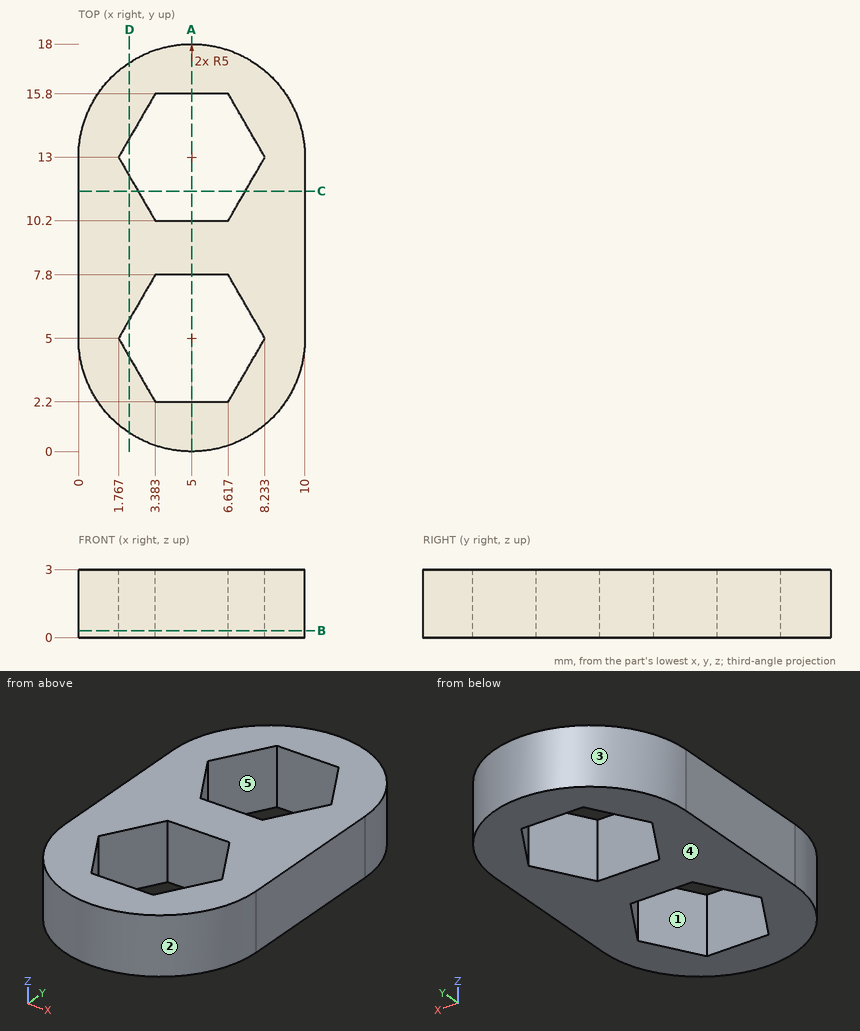
Geometry: see drawing. Coordinates: mm, zero at the bounding-box minimum. A direction names the side the tool comes from. Give positions to 0.01 mm unless a question says otherwise; leave off trailing zeros. Order: outer loops, then holes, each group sorted by start corner. A loop starts at its lowest first (then second) coordinate and runs counter-clockwise, first axis right, second up. Notation, with made-up numbers: (1, -9) -> (15, -9) arc R5 ccw to (15, 0) -> close; hole circle Ø9 at (-11.75, -2). An arc over 180 degrees is marked (long way). Write each question's results on one line, items separated by ' | '. Start each with the question number.
1) Line query: line 1 (Y direction, x = 5.75, z = 2.3); line 2 (Y direction, x = 6.75, z = 1.6) (1 decimal); line 3 (X direction, y = 4.5, z = 1.2) (1 decimal). Output: solid intervals per line, ascending. Write a range as from..to.
2) Draft query along Y for the marked faces 3, 4 and 5. Return one class per face: pulls with the +Y half, pulls with the -Y half, needs draft (parallel to the pull), parting line crosses it, or undercut.
3) Set-up query: the marked faces 1 and 2. Return all of +Z, -Z, +X, -X, +Y, -Y with unobstructed straight access to the full face (end or side cutting, diameter ignored); none if empty.
4) Section A-A (x = 5). Return loops of the section in (y, z).
5) Section B-B (z = 0.3). Return loops of the section in (x, y), then the cut area to 3 significant figures.
6) Section C-C (y = 11.5). Return loops of the section in (x, z).
7) Section D-D (x = 2.25). Return loops of the section in (y, z) (1 decimal), then the cut area to 3 significant figures.
Calculated:
1) line 1: 0.06..2.2, 7.8..10.2, 15.8..17.94 | line 2: 0.3..2.4, 7.6..10.4, 15.6..17.7 | line 3: 0..2.1, 7.9..10
2) face 3: pulls with the +Y half | face 4: needs draft | face 5: undercut
3) face 1: +Z, -Z | face 2: +Z, -Z, -Y
4) outline: (0, 0) -> (2.2, 0) -> (2.2, 3) -> (0, 3) -> close; (7.8, 0) -> (10.2, 0) -> (10.2, 3) -> (7.8, 3) -> close; (15.8, 0) -> (18, 0) -> (18, 3) -> (15.8, 3) -> close
5) outline: (0, 5) arc R5 ccw to (10, 5) -> (10, 13) arc R5 ccw to (0, 13) -> close; hole (1.77, 5) -> (3.38, 2.2) -> (6.62, 2.2) -> (8.23, 5) -> (6.62, 7.8) -> (3.38, 7.8) -> close; hole (1.77, 13) -> (3.38, 10.2) -> (6.62, 10.2) -> (8.23, 13) -> (6.62, 15.8) -> (3.38, 15.8) -> close | area: 104 mm2
6) outline: (0, 0) -> (2.63, 0) -> (2.63, 3) -> (0, 3) -> close; (7.37, 0) -> (10, 0) -> (10, 3) -> (7.37, 3) -> close
7) outline: (0.8, 0) -> (4.2, 0) -> (4.2, 3) -> (0.8, 3) -> close; (5.8, 0) -> (12.2, 0) -> (12.2, 3) -> (5.8, 3) -> close; (13.8, 0) -> (17.2, 0) -> (17.2, 3) -> (13.8, 3) -> close | area: 39.0 mm2
